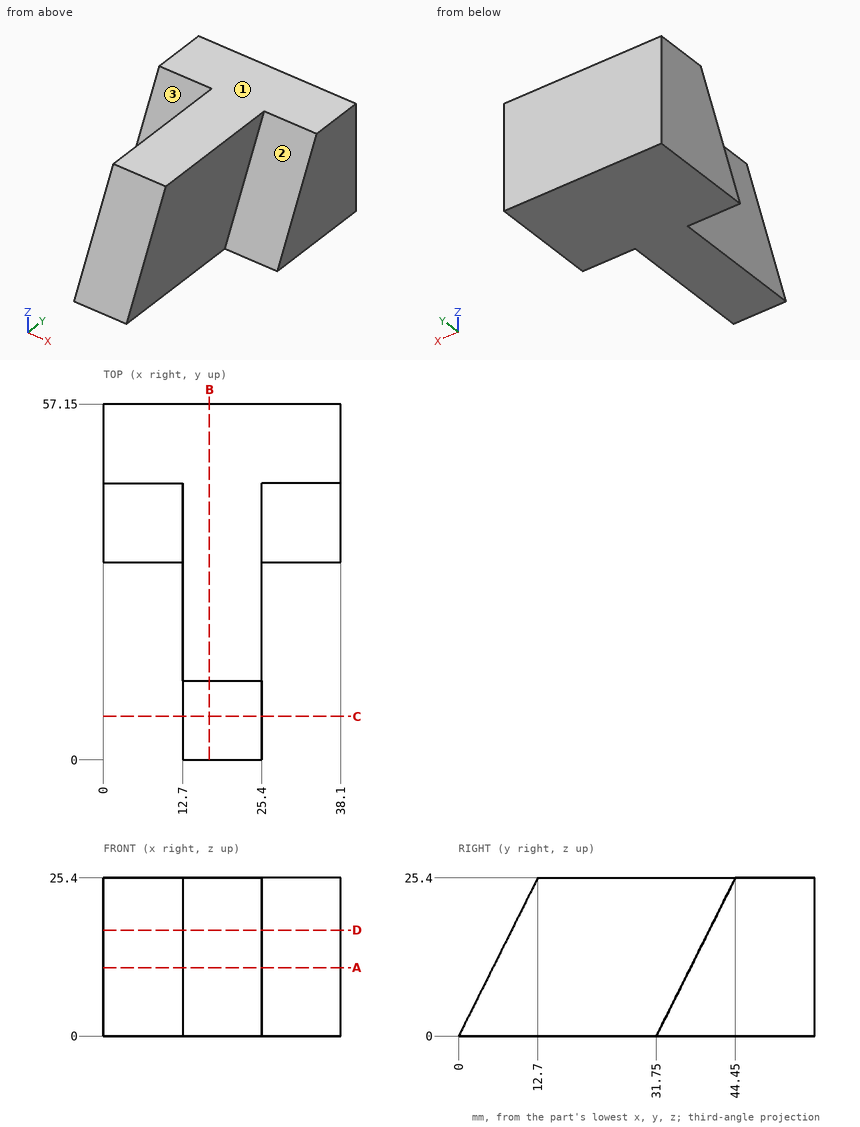
For this review, use the dimensioned drawing (mm, ordinates from the lowest corner) and the shaded views. A direction names the side the tool comes from. Coordinates: 2 decimals unless noted, no trailing zeros. Write each loop counter-clockwise with the first axis right and the second up, starting at its lowest first coordinate (ties: lowest second). Pieces come first, ordered by that corner, then holes. Notation, with made-up numbers: (18, 75.5) -> (61, 75.5) arc R35 ccw to (61, 107.5) -> close; hole circle Ø9 at (-33, -13.75). An arc over 180 degrees is marked (long way). Put each result on its own line as item: value.
Q1. Take a section at D-D, the plane z = 17. State the section outline as (x, y) points, then the cut area to 3 significant figures.
From the geometry:
outline: (0, 40.25) -> (12.7, 40.25) -> (12.7, 8.5) -> (25.4, 8.5) -> (25.4, 40.25) -> (38.1, 40.25) -> (38.1, 57.15) -> (0, 57.15) -> close
area: 1,050 mm2
Q2. Wall thickness on L1, parallel to X at y = 17.5, z = 4; L2, parallel to Y at x = 10.5, z = 22.25 (3 decimals); L3, parallel to Y at x = 17, z = 5: over which ranges is each line inside the solid? List them lowest first.
From the geometry:
L1: x = 12.7 to 25.4
L2: y = 42.875 to 57.15
L3: y = 2.5 to 57.15
Q3. Take a section at B-B, the plane x = 17. State the section outline as (y, z) points.
From the geometry:
outline: (0, 0) -> (57.15, 0) -> (57.15, 25.4) -> (12.7, 25.4) -> close
Q4. Clearance check with flat-ended pins moving along their axes: pin 1 Ø6 at (x, z) = (28, 4.5) entering from -Y; pin 2 Ø5 at (y, z) = (21, 16.5) entering from +X; pin 3 Ø2 at (x, z) = (18.5, 12) entering from -Y. State where each tip first meets the part, or that it passes through.
From the geometry:
pin 1: stops at y = 1.5
pin 2: stops at x = 25.4
pin 3: stops at y = 5.5
Q5. Tool access review of the marked faces 1, 2 and 3: name each direction out of +Z, -Z, +X, -X, +Y, -Y from which nothing blocks a thin tool from reaching the whole face with its end or side.
From the geometry:
face 1: +Z, +X, -X, +Y, -Y
face 2: +Z, +X, -Y
face 3: +Z, -X, -Y
Q6. Take a section at A-A, the plane z = 11. State the section outline as (x, y) points, then the cut area to 3 significant figures.
From the geometry:
outline: (0, 37.25) -> (12.7, 37.25) -> (12.7, 5.5) -> (25.4, 5.5) -> (25.4, 37.25) -> (38.1, 37.25) -> (38.1, 57.15) -> (0, 57.15) -> close
area: 1,160 mm2
Q7. Take a section at C-C, the plane y = 7. State the section outline as (x, z) points.
From the geometry:
outline: (12.7, 0) -> (25.4, 0) -> (25.4, 14) -> (12.7, 14) -> close
